```python
from build123d import *

# Parameters (mm, degrees)
EXTRUDE_1_DEPTH     = 56
SKETCH_3_R          = 7
EXTRUDE_2_DEPTH     = 14
SKETCH_2_R          = 11
SKETCH_2_R_2        = 6
EXTRUDE_3_DEPTH     = 8
SKETCH_8_R          = 6.005758489
CUT_EXTRUDE_1_DEPTH = 10


with BuildPart() as part:
    # 草图1 → 凸台-拉伸1 (new body)
    with BuildSketch(Plane.XY):
        Polygon((-20, 0), (20, 0), (20, -14), (13, -14), (13, -7), (-13, -7), (-13, -14), (-20, -14), align=None)
    extrude(amount=-EXTRUDE_1_DEPTH)

    # 草图3 → 凸台-拉伸2 (add)
    with BuildSketch(Plane(origin=(0, 0, -56), x_dir=(-1, 0, 0), z_dir=(0, 0, -1))):
        with BuildLine():
            ThreePointArc((13.678424719, 28.98340363), (0, 40), (-13.678424719, 28.98340363))
            Line((-13.678424719, 28.98340363), (-20, 0))
            Line((-20, 0), (20, 0))
            Line((20, 0), (13.678424719, 28.98340363))
        make_face()
        with Locations((0, 26)):
            Circle(SKETCH_3_R, mode=Mode.SUBTRACT)
    extrude(amount=-EXTRUDE_2_DEPTH)

    # 草图2 → 凸台-拉伸3 (add)
    with BuildSketch(Plane(origin=(0, 0, 0), x_dir=(1, 0, 0), z_dir=(0, 1, 0))):
        with Locations(Location((0, 20, 0), (0, 0, 270))):
            Circle(SKETCH_2_R)
        with Locations(Location((0, 20, 0), (0, 0, 270))):
            Circle(SKETCH_2_R_2, mode=Mode.SUBTRACT)
    extrude(amount=EXTRUDE_3_DEPTH)

    # 草图8 → 切除-拉伸1 (cut)
    with BuildSketch(Plane(origin=(0, 0, 0), x_dir=(1, 0, 0), z_dir=(0, 1, 0))):
        with Locations(Location((0, 19.994241511, 0), (0, 0, 90.010673287))):
            Circle(SKETCH_8_R)
    extrude(amount=-CUT_EXTRUDE_1_DEPTH, mode=Mode.SUBTRACT)


solid = part.part
```
Check sheet for the modelled part. Datum: model origin and axes. Units: mm. A direction names the side the tool comes from. Round coordinates to 2 decimals unless told otherwise and drop trailing zeros. Write each loop counter-clockwise with the first axis right and the second up, starting at its lowest first coordinate (ties: lowest second). Pieces come first, ordered by that corner, then holes. Notation, with made-up numbers: M -20.75,-32.5 L 32.25,-32.5 A22 ccw 32.25,-11.5 Z; hole C 71.5,3.5 d7. An arc over 180 degrees is marked long. Write item = value, one per line. Start each with the question number.
1. Scan lines: line 1 (X direction, y = -1.5, z = -19.5); line 2 (Y direction, x = 0, z = -46); line 3 (Z direction, x = 0, y = -2). Record each from-to range of solid material in increasing order. Write a range as [from, to].
2. Gauge pin test, flat ends, axial feed: pin 1 (1 mm diameter, centred on x = 15, z = -24.5, fed in from +Y); pin 2 (5 mm diameter, centred on x = -7, y = 29.5, fed in from +Z); pin 3 (13 mm diameter, centred on x = 1.5, z = -16, fed in from -Y). Record the tip position at first contact, or that the pin passes through.
3. Section check C-C, the plane x = 3.5. State how many separate pieces and enclosed holes the cut face has, then the cut area to 3 significant figures.
4. Release check for a two-part mould opening along X. For faces 5 (the flat face through (13, -11, -28)), 6 (the flat face through (-13, -10, -28)), 7 (the cylindrical face through (-4.213, 3.944, -9.839)), 8 (the flat face through (20, -7, -28)) record: pulls with the +X half, pulls with the -X half, needs draft (parallel to the pull), parting line crosses it, or undercut.
5. Section check B-B, the plane y = 22.5. Record the cut outline in (x, z), then the cut area to 3 significant figures.
6. Tool access check on faces 1 (the flat face through (0, 16, -42)), 2 (the cylindrical face through (1.517, 19.166, -49.098)), 3 (the flat face through (0, -7, -28)), 4 (the flat face through (-5, 8, -15)). Record the directions out of +Z, -Z, +X, -X, +Y, -Y that give a thin tool (end or side, any length) a straight path to the whole face; none if there is none.
7. Section check D-D, the plane z = -36. Record the cut outline in (x, y), then the cut area to 3 significant figures.
Results found:
q1.line_1 = [-20, -5.99], [5.99, 20]
q1.line_2 = [-7, 19], [33, 40]
q1.line_3 = [-56, -26], [-13.99, 0]
q2.pin_1 = 0
q2.pin_2 = -42
q2.pin_3 = -7
q3.separate_pieces = 3
q3.enclosed_holes = 0
q3.area = 797 mm^2
q4.face_5 = undercut
q4.face_6 = undercut
q4.face_7 = parting line crosses it
q4.face_8 = pulls with the +X half
q5.outline = M -15.09,-56 L -6.06,-56 L -6.06,-42 L -15.09,-42 Z; M 6.06,-56 L 15.09,-56 L 15.09,-42 L 6.06,-42 Z
q5.area = 253 mm^2
q6.face_1 = +X, -X, +Y
q6.face_2 = +Z, -Z
q6.face_3 = +Z, -Z, -Y
q6.face_4 = +Z, +X, -X, +Y
q7.outline = M -20,-14 L -13,-14 L -13,-7 L 13,-7 L 13,-14 L 20,-14 L 20,0 L -20,0 Z
q7.area = 378 mm^2
